For this review, use the dimensioned drawing (mm, ordinates from the lowest corner) and the shaded views. A direction names the side the tool comes from. Give positions to 0.01 mm unless a question says otherwise; leave off trailing zeros. Order: outer loops, then holes, each group sorted by start corner. A loop starts at its lowest first (then second) coordinate and runs counter-clockwise, first axis right, second up. Notation, with made-up numbers: (24, 85.25) - (70, 85.25) arc R21 ccw to (70, 90.25) - close; hole circle Ø4 at (81, 78.25). An arc over 180 degrees is marked (long way). Use a Markdown table: item, result. Add a question column.
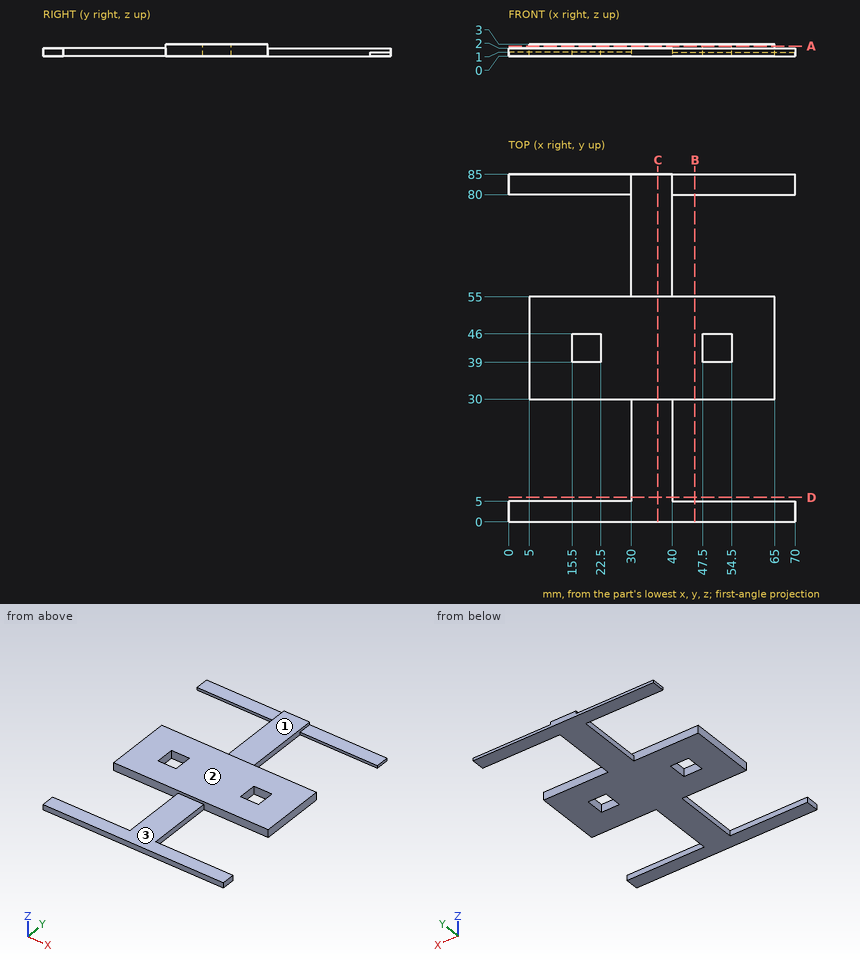
Q1. We need section B-B (x = 45.5). Write out the cut boundary in (y, z).
Q2. Wall thickness on probe 1 along Y at (x, z) = (50.5, 0.1); probe 2 along Y at (x, z) = (58, 0.85); probe 3 along Y at (x, z) = (20.5, 1.4): over which ranges is each line inside the solid? List them lowest first.
Q3. We need section C-C (x = 36.5). Write out the cut boundary in (y, z).
Q4. We need section A-A (z = 2.5). Write out the cut boundary in (x, y), plus the area to 3 significant figures.
Q5. We need section D-D (y = 6). Write out the cut boundary in (x, z), plus the area to 3 significant figures.
Q6. Machinability: for the marked faces 1, 2 and 3, which of the approach directions +Z, -Z, +X, -X, +Y, -Y give a long, thin tool a straight path to every point of the face, cutting with its end or side? Answer none if there is none.
Q7. Clearance check with flat-ended pins moving along their axes: P1, Ø1.5, axis at y = 22.5, z = 1, coming from the -X side; P2, Ø9, axis at x = 30.5, y = 11.5, coming from the +Z side; P3, Ø1.5, axis at x = 9.5, y = 83, coming from the +Z side. State where each tip first meets the part, or that it passes through.
Here are the results:
| question | item | result |
|---|---|---|
| 1 | outline | (0, 0) - (5, 0) - (5, 2) - (0, 2) - close; (30, 0) - (55, 0) - (55, 3) - (30, 3) - close; (80, 0) - (85, 0) - (85, 1) - (80, 1) - close |
| 2 | probe 1 | 0 to 5, 30 to 39, 46 to 55, 80 to 85 |
| 2 | probe 2 | 0 to 5, 30 to 55, 80 to 85 |
| 2 | probe 3 | 0 to 5, 30 to 39, 46 to 55 |
| 3 | outline | (0, 0) - (85, 0) - (85, 2) - (55, 2) - (55, 3) - (30, 3) - (30, 2) - (0, 2) - close |
| 4 | outline | (5, 30) - (65, 30) - (65, 55) - (5, 55) - close; hole (15.5, 39) - (22.5, 39) - (22.5, 46) - (15.5, 46) - close; hole (47.5, 39) - (54.5, 39) - (54.5, 46) - (47.5, 46) - close |
| 4 | area | 1,400 mm2 |
| 5 | outline | (30, 0) - (40, 0) - (40, 2) - (30, 2) - close |
| 5 | area | 20.0 mm2 |
| 6 | face 1 | +Z, +X, -X, +Y |
| 6 | face 2 | +Z, +X, -X, +Y, -Y |
| 6 | face 3 | +Z, +X, -X, -Y |
| 7 | P1 | x = 30 |
| 7 | P2 | z = 2 |
| 7 | P3 | z = 1 |
